Design review of the part shown in the three views and the two pictorial views. Dimensions are in mm from the part's minimum x, y and z. Give positions to 0.01 mm unless a question says otherwise; leave off trailing zeros. Write each loop counter-clockwise with the first axis right and the second up, starting at its lowest first coordinate (ties: lowest second). Pieces come first, ordered by that corner, then holes.
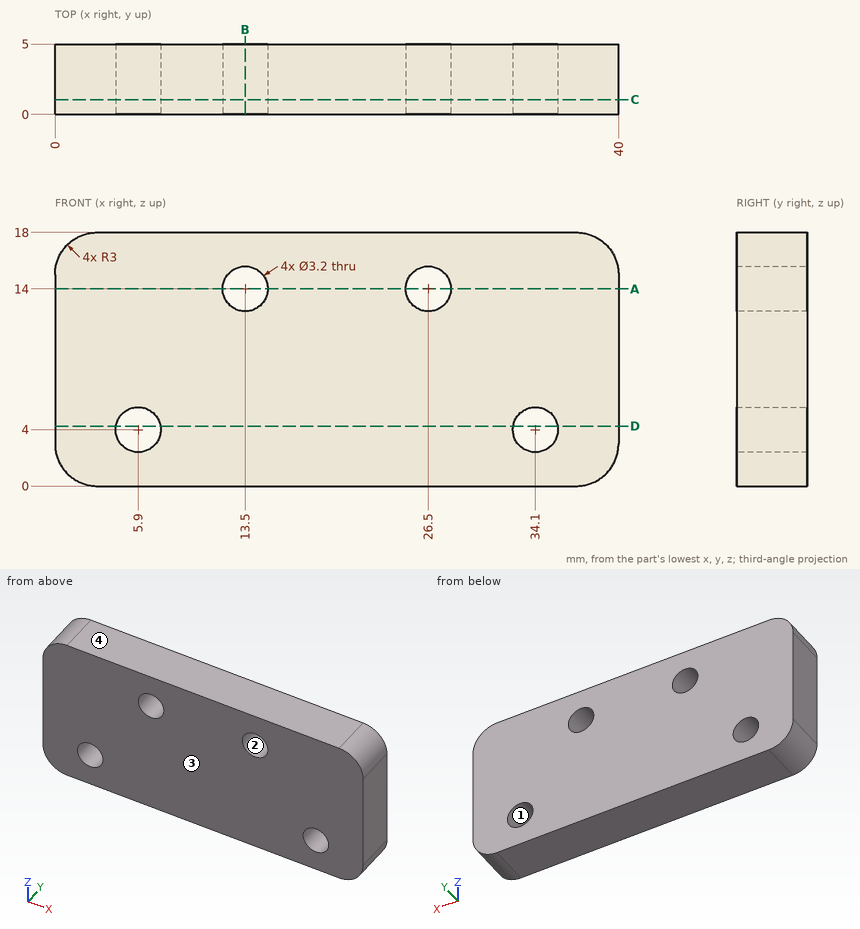
(1) Consider section C-C, the plane y = 1.05. Give the boundary of the cut face in (x, z), then the cut area to 3 significant figures.
Resolved:
outline: (0, 3) arc R3 ccw to (3, 0) - (37, 0) arc R3 ccw to (40, 3) - (40, 15) arc R3 ccw to (37, 18) - (3, 18) arc R3 ccw to (0, 15) - close; hole circle Ø3.2 at (5.9, 4); hole circle Ø3.2 at (13.5, 14); hole circle Ø3.2 at (26.5, 14); hole circle Ø3.2 at (34.1, 4)
area: 680 mm2
(2) To check wall thickness, follow L1, parallel to X at y = 2.15, z = 4; L2, parallel to X at y = 3, z = 14; L3, parallel to Z at x = 14, y = 0.65. State the ranges of each line that lie inside material, in increasing order.
Resolved:
L1: x = 0 to 4.3, 7.5 to 32.5, 35.7 to 40
L2: x = 0 to 11.9, 15.1 to 24.9, 28.1 to 40
L3: z = 0 to 12.48, 15.52 to 18
(3) Consider section A-A, the plane z = 14. Give the boundary of the cut face in (x, y), then the cut area to 3 significant figures.
Resolved:
outline: (0, 0) - (11.9, 0) - (11.9, 5) - (0, 5) - close; (15.1, 0) - (24.9, 0) - (24.9, 5) - (15.1, 5) - close; (28.1, 0) - (40, 0) - (40, 5) - (28.1, 5) - close
area: 168 mm2
(4) Clearance check with flat-ended pins moving along their axes: P1, Ø3, axis at y = 3.5, z = 10, coming from the -X side; P2, Ø2.5, axis at x = 26.5, z = 14, coming from the +Y side. State where each tip first meets the part, or that it passes through.
Resolved:
P1: stops at x = 0
P2: passes through
(5) Mouldability with a two-part tool opening along Z and no side actions: class the marked faces 1, 2, 3 and 4 as pulls with the +Z half, pulls with the -Z half, needs draft (parallel to the pull), parting line crosses it, or undercut.
Resolved:
face 1: undercut
face 2: undercut
face 3: needs draft
face 4: pulls with the +Z half
(6) Consider section D-D, the plane z = 4.25. Give the boundary of the cut face in (x, y), then the cut area to 3 significant figures.
Resolved:
outline: (0, 0) - (4.32, 0) - (4.32, 5) - (0, 5) - close; (7.48, 0) - (32.52, 0) - (32.52, 5) - (7.48, 5) - close; (35.68, 0) - (40, 0) - (40, 5) - (35.68, 5) - close
area: 168 mm2
(7) Consider section B-B, the plane x = 13.5. Give the boundary of the cut face in (y, z), then the cut area to 3 significant figures.
Resolved:
outline: (0, 0) - (5, 0) - (5, 12.4) - (0, 12.4) - close; (0, 15.6) - (5, 15.6) - (5, 18) - (0, 18) - close
area: 74.0 mm2
